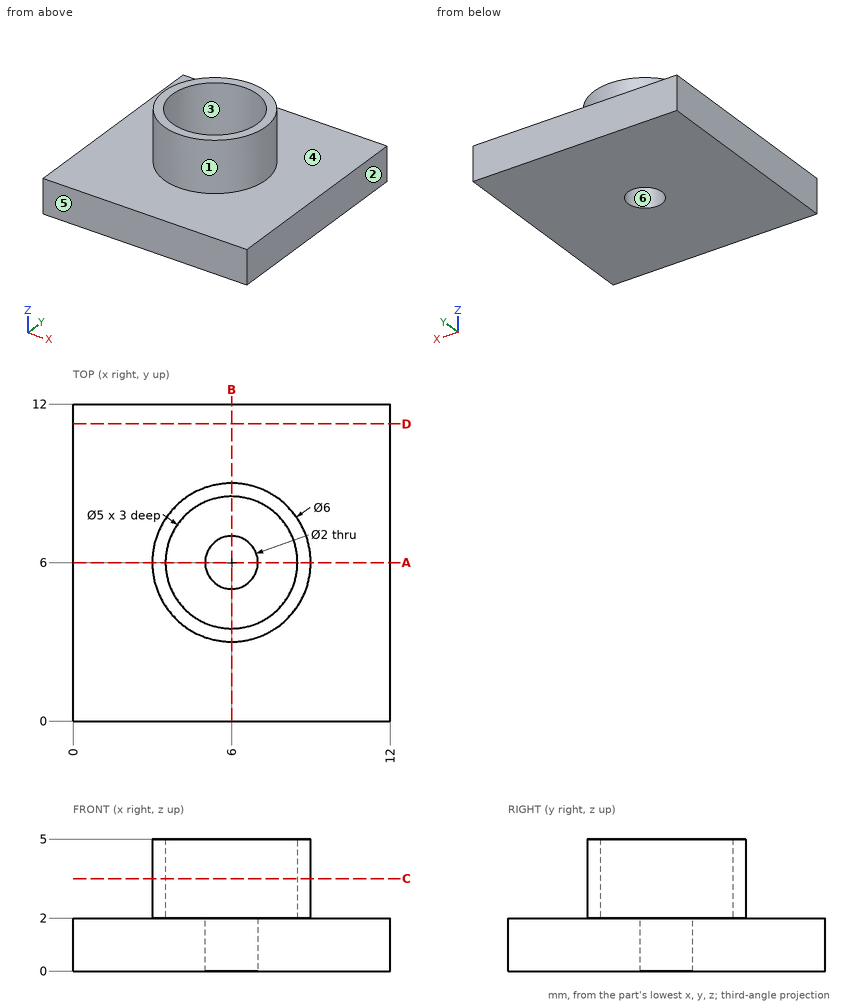
Part print with two shaded views. Sizes in mm from the minimum x, y, z corner. A direction names the side the tool comes from. Coordinates: 2 decimals unless noted, no trailing zeros. Write each loop counter-clockwise with the first axis right and the second up, starting at its lowest first coordinate (ties: lowest second). Pieces come first, ordered by that corner, then holes. Notation, with made-up numbers: (15, 0.25) -> (23, 0.25) arc R23 cw to (23, 29.25) -> close; hole circle Ø10 at (53, 13.25). An arc over 180 degrees is marked (long way). Return JSON: item names as keys, results as strings. Group by question number.
Q1. Cut at D-D, the plane y = 11.25. Give the cut face in (x, z), then the cut area to 3 significant figures.
Q2. Pull direction Y, two halves, no side cores. Call the marked faces 3, 4, 5 and 6: released by +Y, released by -Y, zero draft, split by the parting line, or undercut.
Q3. Drill centre lines: line 1 (Y direction, x = 6, z = 3.25); line 2 (Y direction, x = 6, z = 0.85); line 3 (Z direction, x = 9, y = 2.25). Where is each one in solid material? Low to high.
Q4. Cut at C-C, the plane z = 3.5. Give the cut face in (x, y), then the cut area to 3 significant figures.
Q5. Cut at A-A, the plane y = 6. Give the cut face in (x, z), then the cut area to 3 significant figures.
Q6. Which spindle directions (+Z, -Z, +X, -X, +Y, -Y) get a long thin tool onto all of the face, cutting with end or side? Do the marked faces 1 and 2. Say none if no direction does.
Returned:
{
 "1": {"outline": "(0, 0) -> (12, 0) -> (12, 2) -> (0, 2) -> close", "area": "24.0 mm2"},
 "2": {"face 3": "undercut", "face 4": "zero draft", "face 5": "released by -Y", "face 6": "undercut"},
 "3": {"line 1": "y = 3 to 3.5, 8.5 to 9", "line 2": "y = 0 to 5, 7 to 12", "line 3": "z = 0 to 2"},
 "4": {"outline": "circle Ø6 at (6, 6); hole circle Ø5 at (6, 6)", "area": "8.64 mm2"},
 "5": {"outline": "(0, 0) -> (5, 0) -> (5, 2) -> (3.5, 2) -> (3.5, 5) -> (3, 5) -> (3, 2) -> (0, 2) -> close; (7, 0) -> (12, 0) -> (12, 2) -> (9, 2) -> (9, 5) -> (8.5, 5) -> (8.5, 2) -> (7, 2) -> close", "area": "23.0 mm2"},
 "6": {"face 1": "+Z", "face 2": "+Z, -Z, +X, +Y, -Y"}
}
